from build123d import *

# Parameters (mm, degrees)
SKETCH2_R               = 4
CUT_EXTRUDE1_DEPTH      = 12.5
CHAMFER1_SIZE           = 0.5
CHAMFER2_SIZE           = 0.25
M3_5X0_6_TAPPED_HOLE1_D = 2.9


with BuildPart() as part:
    # Sketch1 → Revolve1 (revolve)
    with BuildSketch(Plane(origin=(0, 0, 0), x_dir=(0, 0, -1), z_dir=(1, 0, 0))):
        Polygon((-5.75, 0), (-5.75, 5), (-1.75, 5), (-1.75, 11), (1.75, 11), (1.75, 5), (5.75, 5), (5.75, 0), align=None)
    revolve(axis=Axis((0, 0, 5.75), (0, 0, -1)))

    # Sketch2 → Cut-Extrude1 (cut, through all)
    with BuildSketch(Plane.XY.offset(5.75)):
        Circle(SKETCH2_R)
    extrude(amount=-CUT_EXTRUDE1_DEPTH, mode=Mode.SUBTRACT)

    # Chamfer1
    chamfer1_edges = [part.edges().sort_by_distance(p)[0] for p in [
        (0, -5, -5.75),
        (0, -5, 5.75),
    ]]
    chamfer(chamfer1_edges, length=CHAMFER1_SIZE)

    # Chamfer2
    chamfer2_edges = [part.edges().sort_by_distance(p)[0] for p in [
        (0, -11, -1.75),
        (0, -11, 1.75),
    ]]
    chamfer(chamfer2_edges, length=CHAMFER2_SIZE)

    # M3.5x0.6 Tapped Hole1 (through all)
    with Locations(Plane.XY.offset(1.75)):
        with Locations((-5.75, 5.75), (5.75, 5.75), (5.75, -5.75), (-5.75, -5.75)):
            Hole(M3_5X0_6_TAPPED_HOLE1_D / 2)


solid = part.part
CAD build for the part. Positions are in the model's coordinates, mm. A direction names the side the tool comes from. Give positions to 0.01 mm unless a question says otherwise; leave off trailing zeros. Order: outer loops, then holes, each group sorted by start corner. A loop starts at its lowest first (then second) coordinate and runs counter-clockwise, first axis right, second up. Notation, with made-up numbers: (-27, 3) - (-6, 3) arc R8 ccw to (-6, 12) - close; hole circle Ø3 at (30.25, -4). An arc over 180 degrees is marked (long way). Write each question's results on one line, items separated by ' | '.
1. 3-axis set-ups, long thin cutter, end or side, ignore diameter. For faces 4 (the face through (-4.88, -1.08, -3.52)), 5 (the face through (-5, -2, 1.75)), 6 (the face through (-4.3, 5.8, 0)): which of +Z, -Z, +X, -X, +Y, -Y reach the whole face in a straight line?
Calculated:
face 4: -Z | face 5: +Z | face 6: +Z, -Z
2. Saw through at A-A on x = 0. List the corners of the cut face in (y, z), and give its area (3 significant figures).
Calculated:
outline: (-11, -1.5) - (-10.75, -1.75) - (-5, -1.75) - (-5, -5.25) - (-4.5, -5.75) - (-4, -5.75) - (-4, 5.75) - (-4.5, 5.75) - (-5, 5.25) - (-5, 1.75) - (-10.75, 1.75) - (-11, 1.5) - close; (4, -5.75) - (4.5, -5.75) - (5, -5.25) - (5, -1.75) - (10.75, -1.75) - (11, -1.5) - (11, 1.5) - (10.75, 1.75) - (5, 1.75) - (5, 5.25) - (4.5, 5.75) - (4, 5.75) - close | area: 64.4 mm2
3. Pull direction X, two halves, no side cores. Call faces 1 (the face through (7.2, -5.7, 0)), 2 (the face through (-3, 3, 5.75)), 3 (the face through (-4.88, -1.08, 3.48)): released by +X, released by -X, zero draft, split by the parting line, or undercut.
Calculated:
face 1: undercut | face 2: zero draft | face 3: split by the parting line
4. Saw through at C-C on z = -0.75. List the corners of the cut face in (x, y).
Calculated:
outline: circle Ø22 at (0, 0); hole circle Ø2.9 at (-5.75, -5.75); hole circle Ø2.9 at (-5.75, 5.75); hole circle Ø8 at (0, 0); hole circle Ø2.9 at (5.75, -5.75); hole circle Ø2.9 at (5.75, 5.75)
5. Saw through at D-D on z = 3.75. List the corners of the cut face in (x, y), and give its area (3 significant figures).
Calculated:
outline: circle Ø10 at (0, 0); hole circle Ø8 at (0, 0) | area: 28.3 mm2
6. Probe L1, parallel to Y at x = 5.75, z = -1; L2, parallel to Z at x = -2, y = 8.5; L3, parallel to Y at x = 3.5, z = -4. List the from-to ranges inside material, lowest first. Write a range as from..to.
Calculated:
L1: y = -9.38..-7.2, -4.3..4.3, 7.2..9.38 | L2: z = -1.75..1.75 | L3: y = -3.57..-1.94, 1.94..3.57
7. Pin check, flat tips, straight feed: pin 1 (5 mm diameter, centred on x = 4.5, z = 4.5, fed in from +Y); pin 2 (4 mm diameter, centred on x = 5.75, y = -5.75, fed in from -Z); pin 3 (4 mm diameter, centred on x = -6, z = -1, fed in from -Y); pin 4 (4 mm diameter, centred on x = 1, y = 0, fed in from -Z) (3 decimals). Stop position of each tip, or through.
Calculated:
pin 1: stops at y = 4.58 | pin 2: stops at z = -1.75 | pin 3: stops at y = -10.25 | pin 4: passes through
